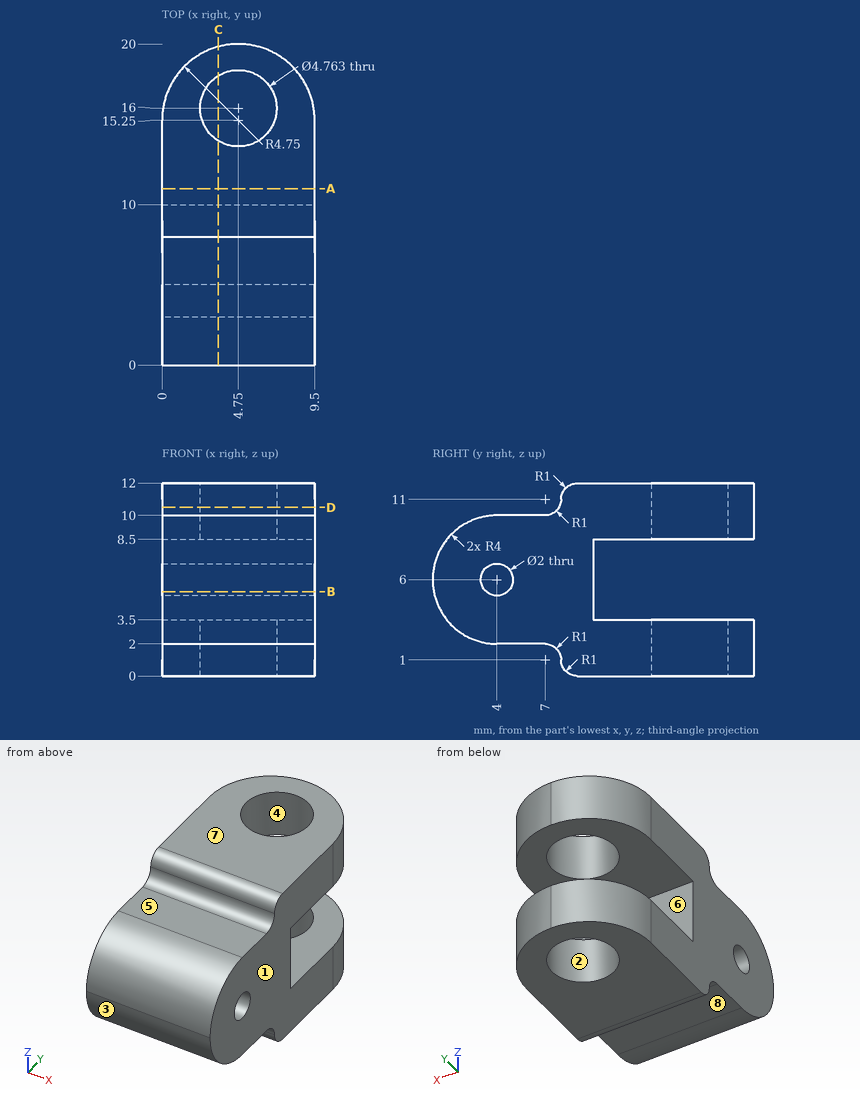
Geometry: see drawing. Coordinates: mm, zero at the bounding-box minimum. A direction names the side the tool comes from. Give positions to 0.01 mm unless a question says otherwise; leave off trailing zeros. Loops run counter-clockwise (first coordinate to the right, second up) from the corner with the lowest first, then second, coordinate; pieces in that order, holes last. Notation, with made-up numbers: (14, 78) - (28, 78) arc R20 cw to (28, 115) - close; hole circle Ø4 at (9.5, 41.5). An arc over 180 degrees is marked (long way). Answer as CSV lines item,"result". Start each with the question number.
1. Section B-B, the plane z = 5.25. Return loops of the section in (x, y).
2. Draft query along X for the marked faces 1, 2 and 3. Return one class per face: released by +X, released by -X, zero draft, split by the parting line, or undercut.
3. Section C-C, the plane x = 3.5. Give the number of separate pieces and of enclosed holes in the cut face.
4. Ray query, L1, parallel to Z at x = 2.75, y = 14; L2, parallel to Y at x = 6.25, z = 6; L3, parallel to Y at x = 4, z = 1.75. Return the intervals inside material, ascending.
5. Pin query (flat end, axial travel): P1, Ø4, axis at x = 4.75, y = 16, coming from the -Z side; P2, Ø2, axis at x = 2.5, z = 2, coming from the +Y side; P3, Ø3, axis at x = 4, z = 4, coming from the -Y side; P4, Ø3.5, axis at x = 7, y = 5, coming from the -Z side. Return the tip coordinate at first contact, or that it passes through.
6. Section A-A, the plane y = 11. Return loops of the section in (x, z).
7. Reachability of the marked faces 4, 5, 6, 7 and 8 from +Z, -Z, +X, -X, +Y, -Y: full face, straight path, thin tool, end or side. Return the list, or none.
8. Section D-D, the plane z = 10.5. Return loops of the section in (x, y).
Answers:
1,outline,"(0, 0.07) - (9.5, 0.07) - (9.5, 3.34) - (0, 3.34) - close; (0, 4.66) - (9.5, 4.66) - (9.5, 10) - (0, 10) - close"
2,face 1,"released by +X"
2,face 2,"undercut"
2,face 3,"zero draft"
3,separate pieces,"3"
3,enclosed holes,"1"
4,L1,"z = 0 to 3.5, 8.5 to 12"
4,L2,"y = 0 to 3, 5 to 10"
4,L3,"y = 7.66 to 13.74, 18.26 to 19.94"
5,P1,"passes through"
5,P2,"stops at y = 19.83"
5,P3,"stops at y = 0.03"
5,P4,"stops at z = 2"
6,outline,"(0, 0) - (9.5, 0) - (9.5, 3.5) - (0, 3.5) - close; (0, 8.5) - (9.5, 8.5) - (9.5, 12) - (0, 12) - close"
7,face 4,"+Z, -Z"
7,face 5,"+Z, +X, -X, -Y"
7,face 6,"+X, -X, +Y"
7,face 7,"+Z, +X, -X, +Y, -Y"
7,face 8,"-Z, +X, -X, -Y"
8,outline,"(0, 7.87) - (9.5, 7.87) - (9.5, 15.25) arc R4.75 ccw to (0, 15.25) - close; hole circle Ø4.76 at (4.75, 16)"
